The listing builds one solid part. Answer for the finished solid, in the listing's coordinates (mm). A direction names the side the tool comes from. Round coordinates to 2 decimals unless told otherwise and drop trailing zeros. Write each loop counter-clockwise with the first axis right and the second up, starting at its lowest first coordinate (ties: lowest second). Pieces come first, ordered by that corner, then holes. Notation, with made-up numbers: (61, 8) - (74, 8) arc R12 ccw to (74, 18) - close; hole circle Ø4 at (-30.75, -12). An arc over 180 degrees is marked (long way). Return JSON: item names as keys, results as strings. Group by question number.
from build123d import *

# Parameters (mm, degrees)
SKETCH1_W           = 50.8
SKETCH1_H           = 76.2
BOSS_EXTRUDE1_DEPTH = 25.4
SKETCH2_W           = 44.45
SKETCH2_H           = 19.05
CUT_EXTRUDE1_DEPTH  = 96.038097624
SKETCH3_R           = 14.2875
CUT_EXTRUDE2_DEPTH  = 3.048


with BuildPart() as part:
    # Sketch1 → Boss-Extrude1 (new body)
    with BuildSketch(Plane.XY):
        with Locations((25.4, 38.1)):
            Rectangle(SKETCH1_W, SKETCH1_H)
    extrude(amount=BOSS_EXTRUDE1_DEPTH)

    # Sketch2 → Cut-Extrude1 (cut, through all)
    with BuildSketch(Plane.XZ):
        with Locations((25.4, 12.7)):
            Rectangle(SKETCH2_W, SKETCH2_H)
    extrude(amount=-CUT_EXTRUDE1_DEPTH, mode=Mode.SUBTRACT)

    # Sketch3 → Cut-Extrude2 (cut)
    with BuildSketch(Plane.XY.offset(25.4)):
        with Locations((25.4, 57.15)):
            Circle(SKETCH3_R)
    extrude(amount=-CUT_EXTRUDE2_DEPTH, mode=Mode.SUBTRACT)


solid = part.part
(1) Find section B-B (x = 25.4). Write down the section's boundary in (y, z) (1 decimal), plus the area to 3 significant figures.
(2) For faces 1 (the flat face through (25, 38, 22.225)), 2 (the cylindrical face through (14.06, 48.46, 23.9)), 3 (the flat face through (50.8, 38, 13)), determine the directions among +Z, -Z, +X, -X, +Y, -Y from which every point of the face is accessible in a straight line to the end or side of a thin tool.
(3) Find section D-D (x = 7). Write down the section's boundary in (y, z) (3 decimals), plus the area to 3 significant figures.
(4) A flat-ended cylindrical pin translates along its axis: pin 1 (5 mm diameter, centred on x = 33.5, y = 61.5, fed in from +Z). Find the tip coordinate at first contact, or state that the pin passes through.
(5) Find section C-C (z = 19). Write down the section's boundary in (x, y) (3 decimals).
(6) Find section A-A (y = 57.15). Write down the section's boundary in (x, z) (1 decimal).
(7) Determine the mould class of faces 4 (the flat face through (25, 39, 25.4)), 5 (the flat face through (47.625, 38, 13)), 6 (the flat face through (0, 38, 13)) for opening direction Z: +Z half, -Z half, draft (parallel to the pull), parting line (faces both ways), or undercut.
(8) Consider line 1 (Z direction, x = 46, y = 72) (3 decimals); line 2 (X direction, y = 25.5, z = 4.75) (3 decimals); line 3 (Y direction, x = 25.4, z = 23.45). Determine where each line is inside the solid, lowest interval first.
Check sheet entries:
{
 "1": {"outline": "(0, 0) - (76.2, 0) - (76.2, 3.2) - (0, 3.2) - close; (0, 22.2) - (76.2, 22.2) - (76.2, 25.4) - (71.4, 25.4) - (71.4, 22.4) - (42.9, 22.4) - (42.9, 25.4) - (0, 25.4) - close", "area": "397 mm^2"},
 "2": {"face 1": "+Y, -Y", "face 2": "+Z", "face 3": "+Z, -Z, +X, +Y, -Y"},
 "3": {"outline": "(0, 0) - (76.2, 0) - (76.2, 3.175) - (0, 3.175) - close; (0, 22.225) - (76.2, 22.225) - (76.2, 25.4) - (0, 25.4) - close", "area": "484 mm^2"},
 "4": {"pin 1": "stops at z = 22.35"},
 "5": {"outline": "(0, 0) - (3.175, 0) - (3.175, 76.2) - (0, 76.2) - close; (47.625, 0) - (50.8, 0) - (50.8, 76.2) - (47.625, 76.2) - close"},
 "6": {"outline": "(0, 0) - (50.8, 0) - (50.8, 25.4) - (39.7, 25.4) - (39.7, 22.4) - (11.1, 22.4) - (11.1, 25.4) - (0, 25.4) - close; hole (3.2, 3.2) - (47.6, 3.2) - (47.6, 22.2) - (3.2, 22.2) - close"},
 "7": {"face 4": "+Z half", "face 5": "undercut", "face 6": "draft"},
 "8": {"line 1": "z = 0 to 3.175, 22.225 to 25.4", "line 2": "x = 0 to 3.175, 47.625 to 50.8", "line 3": "y = 0 to 42.86, 71.44 to 76.2"}
}
